Can you work these out from the model? Positions are in its coordinate system, mm. Give positions to 0.01 mm unless a question says otherwise; leave off trailing zeros. Loops run counter-clockwise (first coordinate to the right, second up) from the corner with the lowest first, then second, coordinate; pieces in that order, holes last. Notation, with made-up numbers: (-22.5, 15.5) -> (21.5, 15.5) arc R26 cw to (21.5, 38.5) -> close; hole circle Ø3 at (5.5, -39.75). An arc over 180 degrees is marked (long way). One line per question, with ' | ' between items.
from build123d import *

# Parameters (mm, degrees)
CONG_1_R = 1


with BuildPart() as part:
    # Esquisse1 → Base-Révolution (revolve)
    with BuildSketch(Plane.XY, mode=Mode.PRIVATE) as base_r_volution_sk:
        with BuildLine():
            Line((0, 11.5), (0, 15))
            Line((0, 15), (14, 15))
            Line((14, 15), (14, 11.5))
            Line((14, 11.5), (12.848076211, 11.5))
            ThreePointArc((12.848076211, 11.5), (10.25, 13), (7.651923789, 11.5))
            Line((7.651923789, 11.5), (6.348076211, 11.5))
            ThreePointArc((6.348076211, 11.5), (3.75, 13), (1.151923789, 11.5))
            Line((1.151923789, 11.5), (0, 11.5))
        make_face()
    revolve(base_r_volution_sk.sketch.rotate(Axis((0, 0, 0), (1, 0, 0)), 90), axis=Axis((0, 0, 0), (1, 0, 0)))

    # Congé1
    cong_1_edges = [part.edges().sort_by_distance(p)[0] for p in [
        (0, 0, -15),
        (14, 0, -15),
    ]]
    fillet(cong_1_edges, radius=CONG_1_R)


solid = part.part
Q1. If we section it at D-D (z = 12.25): State how many separate pieces and enclosed holes the cut face has, plus the area to 3 significant figures.
Entries:
separate pieces: 1 | enclosed holes: 2 | area: 186 mm²
Q2. For pin 1 Ø4 at (x, z) = (10.5, -10) entering from -Y; pin 2 Ø2 at (x, y) = (6.5, -2) entering from -Z; pin 3 Ø6 at (x, z) = (9, 10.5) entering from -Y, each with a flat end and sliding along its axis, tell me the tip position at first contact or that it passes through.
Entries:
pin 1: y = -12.69 | pin 2: z = -14.97 | pin 3: y = -12.99
Q3. If we section it at C-C (x = 2.5): Write out the boundary of the cut face in (y, z), plus the area to 3 significant figures.
Entries:
outline: circle Ø30 at (0, 0); hole circle Ø25.45 at (0, 0) | area: 198 mm²
Q4. If we section it at A-A (y = 0): Write out the boundary of the cut face in (x, z), plus the area to 3 significant figures.
Entries:
outline: (0, -14) arc R1 ccw to (1, -15) -> (13, -15) arc R1 ccw to (14, -14) -> (14, -11.5) -> (12.85, -11.5) arc R3 cw to (7.65, -11.5) -> (6.35, -11.5) arc R3 cw to (1.15, -11.5) -> (0, -11.5) -> close; (0, 11.5) -> (1.15, 11.5) arc R3 cw to (6.35, 11.5) -> (7.65, 11.5) arc R3 cw to (12.85, 11.5) -> (14, 11.5) -> (14, 14) arc R1 ccw to (13, 15) -> (1, 15) arc R1 ccw to (0, 14) -> close | area: 75.0 mm²
Q5. If I drill on probe 1 along X at (y, z) = (-12, -1.5); probe 2 along Z at (x, y) = (6.5, 2.5); probe 3 along Z at (x, y) = (1.5, 1), over which ranges is the centre line in solid material (lowest first)? Write a range as from..to.
Entries:
probe 1: 0..1.6, 5.9..8.1, 12.4..14 | probe 2: -14.79..-11.22, 11.22..14.79 | probe 3: -14.97..-11.94, 11.94..14.97
Q6. If we mould it in two halves opening along Z, with no side actions, what happens to faces 1 (the face through (7.08, -12.65, 8.06)), 2 (the face through (14, -11.5, 2)), 3 (the face through (7, -11.4, -1.5))? For each: pulls with the +Z half, pulls with the -Z half, needs draft (parallel to the pull), parting line crosses it, or undercut.
Entries:
face 1: parting line crosses it | face 2: needs draft | face 3: undercut
